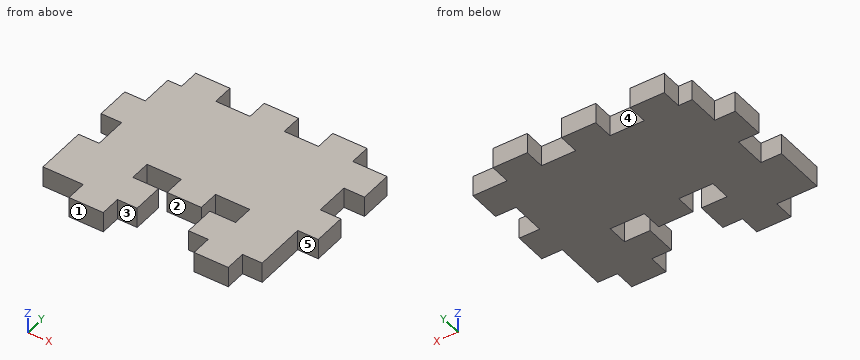
Autodesk Inventor part; units mm, degrees
ref_plane "YZ Plane" through (0, 0, 0) normal (1, 0, 0) x (0, 1, 0)
ref_plane "XZ Plane" through (0, 0, 0) normal (0, 1, 0) x (-1, 0, 0)
ref_plane "XY Plane" through (0, 0, 0) normal (0, 0, 1) x (1, 0, 0)
ref_plane "Work Plane1" through (20, 0, 0) normal (0, 0, 1) x (1, 0, 0)
sketch "Sketch1" plane through (20, 0, 0) normal (0, 0, 1) x (1, 0, 0)
  line L0 (-20, 0) -> (-10, 0)
  line L1 (-10, 0) -> (-10, 6)
  line L2 (-20, 6) -> (-10, 6)
  line L3 (-20, 0) -> (-20, 6)
  line L4 (0, 0) -> (10, 0)
  line L5 (10, 0) -> (10, 6)
  line L6 (0, 6) -> (10, 6)
  line L7 (0, 0) -> (0, 6)
  line L8 (20, 0) -> (30, 0)
  line L9 (30, 0) -> (30, 6)
  line L10 (20, 6) -> (30, 6)
  line L11 (20, 0) -> (20, 6)
  line L12 (-30, 0) -> (-24, 0)
  line L13 (-24, 0) -> (-24, 6)
  line L14 (-30, 6) -> (-24, 6)
  line L15 (-30, 0) -> (-30, 6)
  line L16 (-30, 0) -> (-20, 0)
  line L17 (-10, 0) -> (0, 0)
  line L18 (10, 0) -> (20, 0)
  line L19 (30, 0) -> (40, 0)
  line L20 (40, 0) -> (-24, 0)
  line L21 (-24, 0) -> (-24, -29)
  line L22 (-24, -29) -> (40, -29)
  line L23 (40, -29) -> (40, 0)
  line L24 (-24, -9.5) -> (-30, -9.5)
  line L25 (-30, -9.5) -> (-30, -19.5)
  line L26 (-30, -19.5) -> (-24, -19.5)
  line L27 (-24, -19.5) -> (-24, -9.5)
  line L28 (40, -19.5) -> (34, -19.5)
  line L29 (34, -19.5) -> (34, -9.5)
  line L30 (34, -9.5) -> (40, -9.5)
  line L31 (40, -9.5) -> (40, -19.5)
  line L32 (-24, -14.5) -> (40, -14.5) construction
  line L33 (-20, -29) -> (-10, -29)
  line L34 (-10, -29) -> (-10, -35)
  line L35 (-20, -35) -> (-10, -35)
  line L36 (-20, -29) -> (-20, -35)
  line L37 (0, -29) -> (10, -29)
  line L38 (10, -29) -> (10, -35)
  line L39 (0, -35) -> (10, -35)
  line L40 (0, -29) -> (0, -35)
  line L41 (20, -29) -> (30, -29)
  line L42 (30, -29) -> (30, -35)
  line L43 (20, -35) -> (30, -35)
  line L44 (20, -29) -> (20, -35)
  line L45 (-10, -29) -> (0, -29)
  line L46 (10, -29) -> (20, -29)
  point P0 (-30, -14.5)
  point P1 (34, -14.5)
  dimension "d0" = 29
  dimension "d1" = 6
  dimension "d2" = 10
sketch "Sketch2" plane through (20, 0, 6) normal (0, 0, 1) x (1, 0, 0)
  line L0 (-24, -44) -> (-24, -29)
  line L1 (-18.25, -44) -> (-30, -44)
  line L2 (-2.5, -44) -> (-8.25, -44)
  line L3 (-2.5, -35.5) -> (-2.5, -44)
  line L4 (12, -35) -> (-2, -35)
  line L5 (10, -35) -> (0, -35) construction
  line L6 (5, -35) -> (5, 6) construction
  line L7 (0, 6) -> (10, 6) construction
  line L8 (40, -19.5) -> (34, -19.5)
  line L9 (34, -19.5) -> (34, -9.5)
  line L10 (34, -9.5) -> (40, -9.5)
  line L11 (40, 0) -> (40, -9.5)
  line L12 (30, 0) -> (40, 0)
  line L13 (30, 6) -> (30, 0)
  line L14 (20, 6) -> (30, 6)
  line L15 (20, 0) -> (20, 6)
  line L16 (10, 0) -> (20, 0)
  line L17 (10, 6) -> (10, 0)
  line L18 (0, 6) -> (10, 6)
  line L19 (0, 0) -> (0, 6)
  line L20 (-10, 0) -> (0, 0)
  line L21 (-10, 6) -> (-10, 0)
  line L22 (-20, 6) -> (-10, 6)
  line L23 (-20, 0) -> (-20, 6)
  line L24 (-24, 0) -> (-20, 0)
  line L25 (-24, -9.5) -> (-24, 0)
  line L26 (-30, -9.5) -> (-24, -9.5)
  line L27 (-30, -19.5) -> (-30, -9.5)
  line L28 (-24, -19.5) -> (-30, -19.5)
  line L29 (-24, -29) -> (-24, -19.5)
  line L30 (-20, -29) -> (-24, -29)
  line L31 (-20, -35) -> (-20, -29)
  line L32 (-10, -35) -> (-20, -35)
  line L33 (-10, -29) -> (-10, -35)
  line L34 (0, -29) -> (-10, -29)
  line L35 (0, -35) -> (0, -29)
  line L36 (10, -35) -> (0, -35)
  line L37 (10, -29) -> (10, -35)
  line L38 (20, -29) -> (10, -29)
  line L39 (20, -35) -> (20, -29)
  line L40 (30, -35) -> (20, -35)
  line L41 (30, -29) -> (30, -35)
  line L42 (40, -29) -> (30, -29)
  line L43 (40, -19.5) -> (40, -29)
  line L44 (-2.5, -44) -> (-2.5, -35)
  line L45 (-2.5, -35) -> (0, -35)
  line L46 (-8.25, -50) -> (-18.25, -50)
  line L47 (-18.25, -50) -> (-18.25, -44)
  line L48 (34, -44) -> (34, -29)
  line L49 (12.5, -44) -> (18.25, -44)
  line L50 (12.5, -35.5) -> (12.5, -44)
  line L51 (30, -29) -> (34, -29)
  line L52 (30, -35) -> (30, -29)
  line L53 (20, -35) -> (30, -35)
  line L54 (20, -29) -> (20, -35)
  line L55 (10, -29) -> (20, -29)
  line L56 (10, -35) -> (10, -29)
  line L57 (12.5, -44) -> (12.5, -35)
  line L58 (12.5, -35) -> (10, -35)
  line L59 (18.25, -50) -> (28.25, -50)
  line L60 (28.25, -50) -> (28.25, -44)
  line L61 (28.25, -44) -> (34, -44)
  line L62 (-24, -29) -> (-20, -29)
  line L63 (-20, -35) -> (-20, -29)
  line L64 (-20, -35) -> (-20, -29)
  line L65 (-20, -35) -> (-10, -35)
  line L66 (-10, -35) -> (-10, -29)
  line L67 (0, -29) -> (-10, -29)
  line L68 (0, -29) -> (0, -35)
  line L69 (-8.25, -44) -> (-8.25, -50)
  line L70 (18.25, -50) -> (18.25, -44)
  line L71 (34, -44) -> (34, -29)
  line L72 (28.25, -44) -> (40, -44)
  line L73 (12.5, -44) -> (18.25, -44)
  line L74 (12.5, -35.5) -> (12.5, -44)
  line L75 (30, -29) -> (34, -29)
  line L76 (30, -35) -> (30, -29)
  line L77 (20, -35) -> (30, -35)
  line L78 (20, -29) -> (20, -35)
  line L79 (10, -29) -> (20, -29)
  line L80 (10, -35) -> (10, -29)
  line L81 (12.5, -44) -> (12.5, -35)
  line L82 (12.5, -35) -> (10, -35)
  line L83 (18.25, -50) -> (28.25, -50)
  line L84 (28.25, -50) -> (28.25, -44)
  line L85 (34, -29) -> (30, -29)
  line L86 (30, -35) -> (30, -29)
  line L87 (30, -35) -> (30, -29)
  line L88 (30, -35) -> (20, -35)
  line L89 (20, -35) -> (20, -29)
  line L90 (10, -29) -> (20, -29)
  line L91 (10, -29) -> (10, -35)
  line L92 (18.25, -44) -> (18.25, -50)
  line L93 (-24, -44) -> (-30, -44)
  line L94 (-30, -44) -> (-30, -29)
  line L95 (-30, -29) -> (-24, -29)
  line L96 (-24, -29) -> (-24, -44)
  line L97 (-10, -29) -> (0, -29)
  line L98 (0, -29) -> (0, -35)
  line L99 (0, -35) -> (-10, -35)
  line L100 (-10, -35) -> (-10, -29)
  line L101 (20, -29) -> (10, -29)
  line L102 (10, -29) -> (20, -29)
  line L103 (20, -29) -> (20, -35)
  line L104 (20, -35) -> (10, -35)
  line L105 (10, -35) -> (10, -29)
  line L106 (30, -29) -> (34, -29)
  line L107 (34, -29) -> (34, -35)
  line L108 (34, -35) -> (30, -35)
  line L109 (30, -35) -> (30, -29)
  line L110 (-20, -29) -> (-24, -29)
  line L111 (-24, -29) -> (-24, -35)
  line L112 (-24, -35) -> (-20, -35)
  line L113 (-20, -35) -> (-20, -29)
  line L114 (30, -35) -> (20, -35)
  point P0 (-2.5, -49.5)
  point P1 (12.5, -49.5)
  point P2 (12.5, -49.5)
  dimension "d4" = 10
  dimension "d6" = 6
  dimension "d12" = 6
  dimension "d13" = 15
extrude "Plate1" add sketch "Sketch1" along normal blind 6 contours L3 L2 L1 L0 | L0 L17 L4 L18 L8 L19 L23 L30 L29 L28 L22 L21 L16 | L7 L6 L5 L4 | L21 L26 L25 L24 | L11 L10 L9 L8 | L22 L34 L35 L36 | L22 L38 L39 L40 | L22 L42 L43 L44
sheet face with bend "Face2" sketch "Sketch2" thickness 6 toward (0, 0, -1) bend radius 6 contours L1 L94 L95 L0 | L0 L112 L32 L99 L44 L3 L2 L69 L46 L47 L1 | L0 L30 L31 L112 | L104 L40 L108 L48 L61 L60 L59 L70 L49 L50 L57 | L41 L42 L48 L108
bend "Bend1"
equation "\"d12\" = d6"
equation "\"d3\" = Thickness"
equation "\"d7\" = BendRadius"
equation "\"d8\" = BendReliefWidth"
equation "\"d10\" = MinimumRemnant"
equation "\"d9\" = BendReliefDepth"
equation "\"d11\" = TransitionRadius"
equation "\"BendRadius\" = Thickness"
equation "\"BendReliefWidth\" = Thickness"
equation "\"BendReliefDepth\" = 0.5 * Thickness"
equation "\"CornerReliefSize\" = 4 * Thickness"
equation "\"MinimumRemnant\" = 2 * Thickness"
equation "\"TransitionRadius\" = BendRadius"
equation "\"JacobiRadiusSize\" = BendRadius"
equation "\"GapSize\" = Thickness"
properties part number "jotstick behuizing zijkant" material "Wood (Birch)"
Verification items for the finished model (mm, model axes). Face numbers are marked on the shaded views. A direction names the side the tool comes from. Coordinates: 2 decimals unless noted, no trailing zeros. Order: outer loops, then holes, each group sorted by start corner. A loop starts at its lowest first (then second) coordinate and runs counter-clockwise, first axis right, second up.
Item 1: Section check A-A, the plane y = -47. Enter the section's corners in (x, z).
Filled in:
outline: (1.75, 0) - (11.75, 0) - (11.75, 6) - (1.75, 6) - close; (38.25, 0) - (48.25, 0) - (48.25, 6) - (38.25, 6) - close
Item 2: Section check B-B, the plane y = -39.5. Enter the section's corners in (x, z).
Filled in:
outline: (-10, 0) - (17.5, 0) - (17.5, 6) - (-10, 6) - close; (32.5, 0) - (54, 0) - (54, 6) - (32.5, 6) - close
Item 3: Section check C-C, the plane x = 31.5. Enter the section's corners in (y, z).
Filled in:
outline: (-29, 0) - (0, 0) - (0, 6) - (-29, 6) - close
Item 4: Depth check by flat-ended pin: pin 1 (1.8 mm diameter, centred on y = 3, z = 3.5, fed in from +X); pin 2 (1 mm diameter, centred on x = 33, z = 2.5, fed in from -Y); pin 3 (3 mm diameter, centred on x = 12.5, z = 3.5, fed in from +Y). Enter the tip coordinate at first touch or a pass-through.
Filled in:
pin 1: stops at x = 50
pin 2: stops at y = -44
pin 3: stops at y = 0
Item 5: Section check D-D, the plane y = -15. Enter the section's corners in (x, z).
Filled in:
outline: (-10, 0) - (54, 0) - (54, 6) - (-10, 6) - close
Item 6: Release check for a two-part mould opening along X. For the marked faces 1 and 2 record: +X half, -X half, draft (parallel to the pull), parting line (faces both ways), or undercut.
Filled in:
face 1: draft
face 2: undercut
Item 7: Access from +Z, -Z, +X, -X, +Y, -Y to the whole of each face (thin tool, end or side, straight path). Record for the marked faces 3, 4 and 5.
Filled in:
face 3: +Z, -Z, -Y
face 4: +Z, -Z, +Y
face 5: +Z, -Z, +X, -Y
Item 8: Material ranges on L1, parallel to X at y = 3.5, z = 1.4; L2, parallel to X at y = -30.5, z = 1.25; L3, parallel to X at y = -43.5, z = 5.05, recorded low to high.
Filled in:
L1: x = 0 to 10, 20 to 30, 40 to 50
L2: x = -10 to 10, 20 to 30, 40 to 54
L3: x = -10 to 17.5, 32.5 to 54
